```python
from build123d import *

# Parameters (mm, degrees)
SKETCH1_W           = 150
SKETCH1_H           = 65
BOSS_EXTRUDE1_DEPTH = 40
SKETCH2_W           = 143.904
SKETCH2_H           = 58.904
CUT_EXTRUDE1_DEPTH  = 28.4
SKETCH3_R           = 4.33
CUT_EXTRUDE2_DEPTH  = 3.048


with BuildPart() as part:
    # Sketch1 → Boss-Extrude1 (new body)
    with BuildSketch(Plane(origin=(0, 0, 0), x_dir=(1, 0, 0), z_dir=(0, 1, 0))):
        Rectangle(SKETCH1_W, SKETCH1_H)
    extrude(amount=BOSS_EXTRUDE1_DEPTH)

    # Sketch2 → Cut-Extrude1 (cut)
    with BuildSketch(Plane.XZ):
        Rectangle(SKETCH2_W, SKETCH2_H)
    extrude(amount=-CUT_EXTRUDE1_DEPTH, mode=Mode.SUBTRACT)

    # Sketch3 → Cut-Extrude2 (cut)
    with BuildSketch(Plane(origin=(0, 0, -32.5), x_dir=(-1, 0, 0), z_dir=(0, 0, -1))):
        with Locations((38.12, 12.19)):
            Circle(SKETCH3_R)
    extrude(amount=-CUT_EXTRUDE2_DEPTH, mode=Mode.SUBTRACT)


solid = part.part
```
Check sheet for the modelled part. Datum: model origin and axes. Units: mm. A direction names the side the tool comes from. Round coordinates to 2 decimals unless told otherwise and drop trailing zeros. Loops run counter-clockwise (first coordinate to the right, second up) from the corner with the lowest first, then second, coordinate; pieces in that order, holes last. Notation, with made-up numbers: (80.5, 75) - (112.5, 75) arc R32 ccw to (112.5, 112) - close; hole circle Ø4 at (-25.75, 10.25). An arc over 180 degrees is marked (long way). Write item = value, one per line. Start each with the question number.
Q1. Depth check by flat-ended pin: P1, Ø8, axis at x = -32.5, z = 19.5, coming from the -Y side. Enter the tip coordinate at first touch or a pass-through.
Q2. Section check A-A (x = -38.12). Record the boundary of the cut face in (y, z), plus the area to 3 significant figures.
Q3. Section check B-B (y = 21). Record the boundary of the cut face in (x, z).
Q4. Thickness scan on L1, parallel to X at y = 16.5, z = -5; L2, parallel to Z at x = 35, y = 19.5; L3, parallel to X at y = 12, z = -30. Record the ranges inside material, lowest first.
Q5. Section check D-D (y = 12.19). Record the boundary of the cut face in (x, z).
Q6. Access from +Z, -Z, +X, -X, +Y, -Y to the whole of each face (thin tool, end or side, straight path). Record for faces 1 (the face through (-42.25, 13.49, -31)), 2 (the face through (-1, 20, 32.5)), 3 (the face through (-71.952, 14, 0)).
Q7. Section check C-C (z = -25). Record the boundary of the cut face in (x, y), plus the area to 3 significant figures.
Q8. Release check for a two-part mould opening along X. For faces 4 (the face through (-1, 40, 0)), 5 (the face through (-1, 28.4, 0)), 6 (the face through (-75, 20, 0)) record: pulls with the +X half, pulls with the -X half, needs draft (parallel to the pull), parting line crosses it, or undercut.
Derived:
q1.P1 = 28.4
q2.outline = (0, -32.5) - (7.86, -32.5) - (7.86, -29.45) - (0, -29.45) - close; (0, 29.45) - (28.4, 29.45) - (28.4, -29.45) - (16.52, -29.45) - (16.52, -32.5) - (40, -32.5) - (40, 32.5) - (0, 32.5) - close
q2.area = 901 mm^2
q3.outline = (-75, -32.5) - (75, -32.5) - (75, 32.5) - (-75, 32.5) - close; hole (-71.95, -29.45) - (71.95, -29.45) - (71.95, 29.45) - (-71.95, 29.45) - close
q4.L1 = -75 to -71.95, 71.95 to 75
q4.L2 = -32.5 to -29.45, 29.45 to 32.5
q4.L3 = -75 to -42.45, -33.79 to 75
q5.outline = (-75, -32.5) - (-42.45, -32.5) - (-42.45, -29.45) - (-71.95, -29.45) - (-71.95, 29.45) - (71.95, 29.45) - (71.95, -29.45) - (-33.79, -29.45) - (-33.79, -32.5) - (75, -32.5) - (75, 32.5) - (-75, 32.5) - close
q6.face_1 = -Z
q6.face_2 = +Z, +X, -X, +Y, -Y
q6.face_3 = -Y
q7.outline = (-75, 0) - (-71.95, 0) - (-71.95, 28.4) - (71.95, 28.4) - (71.95, 0) - (75, 0) - (75, 40) - (-75, 40) - close
q7.area = 1,910 mm^2
q8.face_4 = needs draft
q8.face_5 = undercut
q8.face_6 = pulls with the -X half
